from build123d import *

# Parameters (mm, degrees)
SKETCH2_R           = 3.9751
SKETCH2_R_2         = 3.2258
BOSS_EXTRUDE1_DEPTH = 12.7
SKETCH3_R           = 6.35
SKETCH3_R_2         = 3.9751
BOSS_EXTRUDE2_DEPTH = 0.79375
CUT_EXTRUDE1_START  = 4.7625
SKETCH4_R           = 6.35
CUT_EXTRUDE1_DEPTH  = 8.14375


with BuildPart() as part:
    # Sketch2 → Boss-Extrude1 (new body)
    with BuildSketch(Plane(origin=(0, 0, 0), x_dir=(1, 0, 0), z_dir=(0, 1, 0))):
        Circle(SKETCH2_R)
        Circle(SKETCH2_R_2, mode=Mode.SUBTRACT)
    extrude(amount=BOSS_EXTRUDE1_DEPTH)

    # Sketch3 → Boss-Extrude2 (add)
    with BuildSketch(Plane(origin=(0, 0, 0), x_dir=(1, 0, 0), z_dir=(0, 1, 0))):
        Circle(SKETCH3_R)
        Circle(SKETCH3_R_2, mode=Mode.SUBTRACT)
    extrude(amount=BOSS_EXTRUDE2_DEPTH)

    # Sketch4 → Cut-Extrude1 (cut, through all)
    with BuildSketch(Plane(origin=(0, 0.79375, 0), x_dir=(1, 0, 0), z_dir=(0, 1, 0)).offset(CUT_EXTRUDE1_START)):
        Circle(SKETCH4_R)
    extrude(amount=CUT_EXTRUDE1_DEPTH, mode=Mode.SUBTRACT)


solid = part.part
For this review, take the finished solid that the model builds, in its own axes (mm). A direction names the side the tool comes from. Round coordinates to 2 decimals unless told otherwise and drop trailing zeros. Order: outer loops, then holes, each group sorted by start corner. A loop starts at its lowest first (then second) coordinate and runs counter-clockwise, first axis right, second up. Notation, with made-up numbers: (32.5, 51.5) -> (45.5, 51.5) arc R9 ccw to (45.5, 64.5) -> close; hole circle Ø7 at (46, -34). An arc over 180 degrees is marked (long way). Write item = value, one per line. Start each with the question number.
1) To check wall thickness, follow line 1 (Z direction, x = 0, y = 3.4); line 2 (Y direction, x = 3, z = 4.25). State the ranges of each line that lie inside material, in increasing order. Write a range as from..to.
2) Insertion check: pin 1 (1.5 mm diameter, centred on x = 2.5, y = 4, fed in from -Z); pin 2 (2 mm diameter, centred on x = -4, z = 2.5, fed in from +Y). Each pin has a flat end and moves straight along its axis. Give the tip position at first contact, or say it passes through.
3) Take a section at A-A on z = 0. State the section outline as (x, y) points, plus the area to 3 significant figures.
4) Take a section at C-C on y = 4.9. State the section outline as (x, z) points.
5) Tool access review of faces 1 (the face through (-1.38, 0.39, 6.2)), 2 (the face through (-0.86, 3.14, 3.88)): name each direction out of +Z, -Z, +X, -X, +Y, -Y from which nothing blocks a thin tool from reaching the whole face with its end or side.
6) Take a section at B-B on x = 0. State the section outline as (y, z) points, plus the area to 3 significant figures.
7) Take a section at D-D on x = 3.5. State the section outline as (y, z) points, plus the area to 3 significant figures.
Verdict:
q1.line_1 = -3.98..-3.23, 3.23..3.98
q1.line_2 = 0..0.79
q2.pin_1 = -3.57
q2.pin_2 = 5.56
q3.outline = (-6.35, 0) -> (-3.23, 0) -> (-3.23, 5.56) -> (-3.98, 5.56) -> (-3.98, 0.79) -> (-6.35, 0.79) -> close; (3.23, 0) -> (6.35, 0) -> (6.35, 0.79) -> (3.98, 0.79) -> (3.98, 5.56) -> (3.23, 5.56) -> close
q3.area = 12.1 mm2
q4.outline = circle Ø7.95 at (0, 0); hole circle Ø6.45 at (0, 0)
q5.face_1 = +Y, -Y
q5.face_2 = +Y
q6.outline = (0, -6.35) -> (0.79, -6.35) -> (0.79, -3.98) -> (5.56, -3.98) -> (5.56, -3.23) -> (0, -3.23) -> close; (0, 3.23) -> (5.56, 3.23) -> (5.56, 3.98) -> (0.79, 3.98) -> (0.79, 6.35) -> (0, 6.35) -> close
q6.area = 12.1 mm2
q7.outline = (0, -5.3) -> (0.79, -5.3) -> (0.79, -1.88) -> (5.56, -1.88) -> (5.56, 1.88) -> (0.79, 1.88) -> (0.79, 5.3) -> (0, 5.3) -> close
q7.area = 26.4 mm2
